Check sheet for the modelled part. Datum: model origin and axes. Units: mm. A direction names the side the tool comes from. Round coordinates to 2 decimals unless told otherwise and drop trailing zeros. Order: outer loops, then holes, each group sorted by start corner. A loop starts at its lowest first (then second) coordinate and runs counter-clockwise, first axis right, second up.
(1) Thickness scan on probe 1 along Y at (x, z) = (-1.25, -1.5); probe 2 along Z at (x, y) = (4.25, -12.25); probe 3 along Z at (x, y) = (-2, -12). Record the ranges inside material, lowest first.
(2) Sectioned sample at B-B, the plane z = 0. Enter the section's corners in (x, y).
(3) Sectioned sample at C-C, the plane y = -3. Enter the section's corners in (x, z) (1 decimal), and give its area (3 significant figures).
(4) Depth check by flat-ended pin: pin 1 (4 mm diameter, centred on x = -2, z = -3, fed in from -Y); pin 2 (3 mm diameter, centred on y = -4, z = 0, fed in from +X); pin 3 (2 mm diameter, centred on x = -1, y = 7.5, fed in from +Z). Enter the tip coordinate at first touch or a pass-through.
(5) Tool access check on faces 1 (the flat face through (0, 11.906, 0)), 2 (the cylindrical face through (-0.34, -0.17, -1.55)). Record the directions out of +Z, -Z, +X, -X, +Y, -Y that give a thin tool (end or side, any length) a straight path to the whole face; none if there is none.
(6) Sectioned sample at A-A, the plane x = 0. Enter the section's corners in (y, z).
```python
from build123d import *

# Parameters (mm, degrees)
F0_R     = 1.5875
F1_DEPTH = 11.90625
F2_R     = 4.7625
F3_DEPTH = 3.175
F4_R     = 2.032


# Not quite as in the source:
# - a length typed as a fraction of an inch, garbled in the dataset ("3 / 203.2 mm" for 3/8 in), is restored


with BuildPart() as f1:
    # F0 (on Front) → F1 (new body, symmetric)
    with BuildSketch(Plane.XZ):
        Circle(F0_R)
    extrude(amount=F1_DEPTH, both=True)

    # F2 (on face) → F3 (join)
    with BuildSketch(Plane.XZ.offset(11.90625)):
        Circle(F2_R)
    extrude(amount=F3_DEPTH)

    # F4
    f4_edges = [f1.edges().sort_by_distance(p)[0] for p in [
        (-4.7625, -15.08125, 0),
    ]]
    fillet(f4_edges, radius=F4_R)


solid = f1.part
```
Derived:
1. probe 1: y = -15.08 to -11.91
1. probe 2: z = -2.15 to 2.15
1. probe 3: z = -4.32 to 4.32
2. outline: (-4.76, -13.05) arc R2.03 ccw to (-2.73, -15.08) - (2.73, -15.08) arc R2.03 ccw to (4.76, -13.05) - (4.76, -11.91) - (1.59, -11.91) - (1.59, 11.91) - (-1.59, 11.91) - (-1.59, -11.91) - (-4.76, -11.91) - close
3. outline: circle Ø3.2 at (0, 0)
3. area: 7.92 mm2
4. pin 1: stops at y = -15.08
4. pin 2: stops at x = 1.59
4. pin 3: stops at z = 1.59
5. face 1: +Z, -Z, +X, -X, +Y
5. face 2: +Y
6. outline: (-15.08, -2.73) arc R2.03 ccw to (-13.05, -4.76) - (-11.91, -4.76) - (-11.91, -1.59) - (11.91, -1.59) - (11.91, 1.59) - (-11.91, 1.59) - (-11.91, 4.76) - (-13.05, 4.76) arc R2.03 ccw to (-15.08, 2.73) - close
